```python
from build123d import *

# Parameters (mm, degrees)
EXTRUDE_1_DEPTH     = 1.8
SKETCH_2_R          = 4.05
CUT_EXTRUDE_1_DEPTH = 1.8


with BuildPart() as part:
    # 草图1 → 凸台-拉伸1 (new body)
    with BuildSketch(Plane.XY):
        with BuildLine():
            Line((-2, 8.94427191), (-2, 9.8))
            ThreePointArc((-2, 9.8), (-1.941421356, 9.941421356), (-1.8, 10))
            Line((-1.8, 10), (1.8, 10))
            ThreePointArc((1.8, 10), (1.941421356, 9.941421356), (2, 9.8))
            Line((2, 9.8), (2, 8.94427191))
            ThreePointArc((2, 8.94427191), (2.522774425, 6.494782167), (4, 4.472135955))
            ThreePointArc((4, 4.472135955), (0, -6), (-4, 4.472135955))
            ThreePointArc((-4, 4.472135955), (-2.522774425, 6.494782167), (-2, 8.94427191))
        make_face()
    extrude(amount=-EXTRUDE_1_DEPTH)

    # 草图2 → 切除-拉伸1 (cut)
    with BuildSketch(Plane.XY):
        Circle(SKETCH_2_R)
    extrude(amount=-CUT_EXTRUDE_1_DEPTH, mode=Mode.SUBTRACT)


solid = part.part
```
Can you work these out from the model? Positions are in its coordinate system, mm. A direction names the side the tool comes from. Give positions to 0.01 mm unless a question says otherwise; leave off trailing zeros. Loops run counter-clockwise (first coordinate to the right, second up) from the corner with the lowest first, then second, coordinate; pieces in that order, holes last. Notation, with made-up numbers: M 88,42.5 L 132,42.5 A12 cw 132,55.5 Z; hole C -15,53 d8. An arc over 180 degrees is marked long. Use CSV: the item, a comma, the result in double quotes. Start each with the question number.
1. If we mould it in two halves opening along Y, with no side actions, what happens to faces 1 (the face through (0, 10, -1)), 2 (the face through (-0.878, -3.954, -0.887)), 3 (the face through (3, 4, -1.8))? For each: released by +Y, released by -Y, zero draft, split by the parting line, or undercut.
2. On a 3-axis mill with a long thin cutter (end or side, diameter ignored), from which of +Z, -Z, +X, -X, +Y, -Y can I reach the whole of each face in a straight line? I mean faces 4 (the face through (-2, 9.4, -0.9)), 5 (the face through (2, 9.4, -0.9)), 6 (the face through (3, 4, 0)). Say none if no direction works.
3. Imagine slicing it at C-C, the plane y = 0. Write out the boundary of the cut face in (x, z).
4. For P1, Ø0.9, axis at y = 9.5, z = -1, coming from the +X side, with a flat end and sliding along its axis, tell me the tip position at first contact or that it passes through.
5. Imagine slicing it at B-B, the plane z = -0.95. Write out the boundary of the cut face in (x, y).
6. Imagine slicing it at A-A, the plane x = 0. Write out the boundary of the cut face in (y, z).
7. If I drill on L1, parallel to Y at x = 0, z = -0.5; L2, parallel to X at y = -1.5, z = -1.1; L3, parallel to X at y = -1.25, z = -1.35, over which ranges is the centre line in solid material (lowest first)?
8. Imagine slicing it at D-D, the plane y = 6.25. Write out the boundary of the cut face in (x, z).
Response values:
1,face 1,"released by +Y"
1,face 2,"undercut"
1,face 3,"zero draft"
2,face 4,"+Z, -Z, -X, +Y"
2,face 5,"+Z, -Z, +X, +Y"
2,face 6,"+Z, +X, -X, +Y, -Y"
3,outline,"M -6,-1.8 L -4.05,-1.8 L -4.05,0 L -6,0 Z; M 4.05,-1.8 L 6,-1.8 L 6,0 L 4.05,0 Z"
4,P1,"x = 2"
5,outline,"M -4,4.47 A6 ccw long 4,4.47 A6 cw 2,8.94 L 2,9.8 A0.2 ccw 1.8,10 L -1.8,10 A0.2 ccw -2,9.8 L -2,8.94 A6 cw Z; hole C 0,0 d8.1"
6,outline,"M -6,-1.8 L -4.05,-1.8 L -4.05,0 L -6,0 Z; M 4.05,-1.8 L 10,-1.8 L 10,0 L 4.05,0 Z"
7,L1,"-6 to -4.05, 4.05 to 10"
7,L2,"-5.81 to -3.76, 3.76 to 5.81"
7,L3,"-5.87 to -3.85, 3.85 to 5.87"
8,outline,"M -2.64,-1.8 L 2.64,-1.8 L 2.64,0 L -2.64,0 Z"
